from build123d import *

# Parameters (mm, degrees)
SKETCH1_R           = 3
SKETCH1_R_2         = 22.175
BOSS_EXTRUDE1_DEPTH = 4
CUT_EXTRUDE1_DEPTH  = 5
SKETCH3_R           = 3.15
BOSS_EXTRUDE2_DEPTH = 4


with BuildPart() as part:
    # Sketch1 → Boss-Extrude1 (new body)
    with BuildSketch(Plane.XY):
        Polygon((0, 36.632796194), (-9.339584462, 32.184793438), (-11.263738257, 27.930920523), (-58.646229282, 26.490266956), (-76.5, 13.335918569), (-76.5, -13.335918569), (-58.646229282, -26.490266956), (-11.263738257, -27.930920523), (-9.339584462, -32.184793438), (0, -36.632796194), (9.339584462, -32.184793438), (11.263738257, -27.930920523), (58.646229282, -26.490266956), (76.5, -13.335918569), (76.5, 13.335918569), (58.646229282, 26.490266956), (11.263738257, 27.930920523), (9.339584462, 32.184793438), align=None)
        with Locations((0, 30)):
            Circle(SKETCH1_R, mode=Mode.SUBTRACT)
        with Locations((-50, 0)):
            Circle(SKETCH1_R_2, mode=Mode.SUBTRACT)
        with Locations((50, 0)):
            Circle(SKETCH1_R_2, mode=Mode.SUBTRACT)
        with Locations((0, -30)):
            Circle(SKETCH1_R, mode=Mode.SUBTRACT)
    extrude(amount=BOSS_EXTRUDE1_DEPTH)

    # Sketch2 → Cut-Extrude1 (cut, through all)
    with BuildSketch(Plane.XY.offset(4)):
        with BuildLine():
            Line((10, 8.25), (-10, 8.25))
            ThreePointArc((-10, 8.25), (-12.828427125, 7.078427125), (-14, 4.25))
            Line((-14, 4.25), (-14, -4.25))
            ThreePointArc((-14, -4.25), (-12.828427125, -7.078427125), (-10, -8.25))
            Line((-10, -8.25), (10, -8.25))
            ThreePointArc((10, -8.25), (12.828427125, -7.078427125), (14, -4.25))
            Line((14, -4.25), (14, 4.25))
            ThreePointArc((14, 4.25), (12.828427125, 7.078427125), (10, 8.25))
        make_face()
    extrude(amount=-CUT_EXTRUDE1_DEPTH, mode=Mode.SUBTRACT)

    # Sketch3 → Boss-Extrude2 (add)
    with BuildSketch(Plane.XY.offset(4)):
        Polygon((-60.436095429, 25.171524645), (-70.470429489, 30.155905977), (-80.018831674, 22.70201384), (-76.5, 13.335918569), align=None)
        with Locations((-73.15, 21.8)):
            Circle(SKETCH3_R, mode=Mode.SUBTRACT)
        Polygon((76.5, 13.335918569), (60.436095429, 25.171524645), (70.470429489, 30.155905977), (80.018831674, 22.70201384), align=None)
        with Locations((73.15, 21.8)):
            Circle(SKETCH3_R, mode=Mode.SUBTRACT)
        Polygon((60.436095429, -25.171524645), (70.470429489, -30.155905977), (80.018831674, -22.70201384), (76.5, -13.335918569), align=None)
        with Locations((73.15, -21.8)):
            Circle(SKETCH3_R, mode=Mode.SUBTRACT)
        Polygon((-76.5, -13.335918569), (-60.436095429, -25.171524645), (-70.470429489, -30.155905977), (-80.018831674, -22.70201384), align=None)
        with Locations((-73.15, -21.8)):
            Circle(SKETCH3_R, mode=Mode.SUBTRACT)
    extrude(amount=-BOSS_EXTRUDE2_DEPTH)


solid = part.part
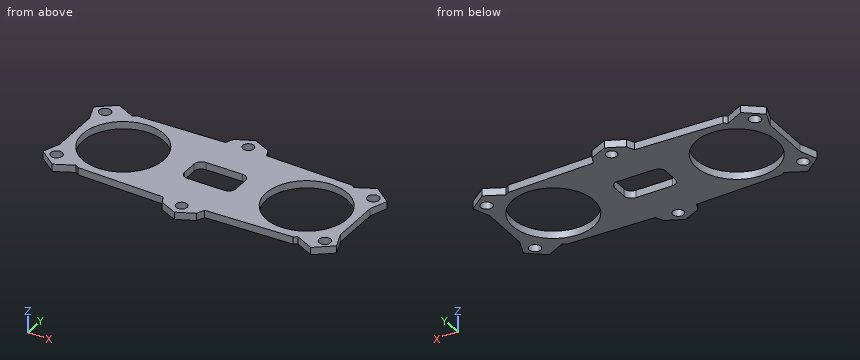
Read the model definition and answer for the solid it produces. Units are mm, in the model's axes. Give positions to 0.01 mm unless a question says otherwise; leave off trailing zeros. Write each loop counter-clockwise with the first axis right and the second up, starting at its lowest first coordinate (ties: lowest second). Pieces come first, ordered by that corner, then holes. Notation, with made-up numbers: (-33.75, -22.75) - (4.25, -22.75) arc R28 ccw to (4.25, 3.25) - close; hole circle Ø6 at (-2.5, -19.5). An arc over 180 degrees is marked (long way). Use CSV: the item, a comma, the result in double quotes. Start each with the question number.
Item 1: The part is cut by section A-A, the plane y = 0. Give the vertices of the cut face in (x, z) (3 decimals).
Item 2: The part is cut by section D-D, the plane x = -68. Give the vertices of the cut face in (y, z), and give its area (3 significant figures).
Item 3: Consider line 1 (Y direction, x = 0, z = 2.05); line 2 (Y direction, x = -73.15, z = 1.75); line 3 (X direction, y = 6.5, z = 0.65). Determine where each line is inside the solid, lowest interval first.
Item 4: Flat-ended cylindrical pins translate along their axes: P1, Ø5.5, axis at x = 73.15, y = -21.8, coming from the +Z side; P2, Ø1.2, axis at x = -2.5, z = 2.5, coming from the +Y side; P3, Ø1.2, axis at y = -6, z = 2, coming from the +X side; P4, Ø1.5, axis at y = 14, z = 2, coming from the -X side. Find the tip coordinate at first contact, or state that the pin passes through.
Item 5: The part is cut by section B-B, the plane x = 35. Give the vertices of the cut face in (y, z), and give its area (3 significant figures).
Item 6: The part is cut by section C-C, the plane z = 2.95. Count the separate pieces of the cut face and the enclosed holes in it, and give its area (3 significant figures).
Taken from the geometry:
1,outline,"(-76.5, 0) - (-72.175, 0) - (-72.175, 4) - (-76.5, 4) - close; (-27.825, 0) - (-14, 0) - (-14, 4) - (-27.825, 4) - close; (14, 0) - (27.825, 0) - (27.825, 4) - (14, 4) - close; (72.175, 0) - (76.5, 0) - (76.5, 4) - (72.175, 4) - close"
2,outline,"(-28.93, 0) - (-12.95, 0) - (-12.95, 4) - (-28.93, 4) - close; (12.95, 0) - (28.93, 0) - (28.93, 4) - (12.95, 4) - close"
2,area,"128 mm2"
3,line 1,"-36.63 to -33, -27 to -8.25, 8.25 to 27, 33 to 36.63"
3,line 2,"-28.06 to -24.95, -18.65 to 18.65, 24.95 to 28.06"
3,line 3,"-76.5 to -71.2, -28.8 to -13.31, 13.31 to 28.8, 71.2 to 76.5"
4,P1,"through"
4,P2,"y = 35.73"
4,P3,"x = 76.5"
4,P4,"x = -77.03"
5,outline,"(-27.21, 0) - (-16.33, 0) - (-16.33, 4) - (-27.21, 4) - close; (16.33, 0) - (27.21, 0) - (27.21, 4) - (16.33, 4) - close"
5,area,"87.0 mm2"
6,separate pieces,"1"
6,enclosed holes,"9"
6,area,"5,010 mm2"
